Here's how the part is built. I have some questions about the finished solid (model axes, mm). A direction names the side the tool comes from. Give positions to 0.01 mm unless a question says otherwise; leave off trailing zeros. Loops run counter-clockwise (first coordinate to the right, second up) from the corner with the lowest first, then second, coordinate; pieces in that order, holes last. Notation, with made-up numbers: (-7, 42) - (46, 42) arc R18 cw to (46, 55) - close; hole circle Ø6 at (35, 70.5). An arc over 180 degrees is marked (long way). Use one line per item in the form item = value.
from build123d import *

# Parameters (mm, degrees)
F0_R     = 2.2923424458
F1_DEPTH = 3


with BuildPart() as f1:
    # F0 (on Top) → F1 (new body)
    with BuildSketch(Plane.XY):
        with BuildLine():
            ThreePointArc((-10.2711248099, 20.5369088401), (-7.4915699128, 20.9637629982), (-4.6818986464, 21.0815648356))
            ThreePointArc((-4.6818986464, 21.0815648356), (-3.8272791749, 22.4288026174), (-3.528424334, 23.9960007114))
            ThreePointArc((-3.528424334, 23.9960007114), (-9.7309143278, 27.7851076735), (-10.2711248099, 20.5369088401))
        make_face()
        with Locations((-7.7870538317, 23.9960007114)):
            Circle(F0_R, mode=Mode.SUBTRACT)
        with BuildLine():
            ThreePointArc((-10.2711248099, 20.5369088401), (-7.3740175906, 19.7574483332), (-4.6818986464, 21.0815648356))
            ThreePointArc((-4.6818986464, 21.0815648356), (-7.4915699128, 20.9637629982), (-10.2711248099, 20.5369088401))
        make_face()
        with BuildLine():
            ThreePointArc((17.6210584616, 7.2744961396), (-14.3609161452, -12.5373076401), (9.5862937371, 16.4779539925))
            ThreePointArc((9.5862937371, 16.4779539925), (2.7986315485, 19.8534789731), (-4.6818986464, 21.0815648356))
            ThreePointArc((-4.6818986464, 21.0815648356), (-7.3740175906, 19.7574483332), (-10.2711248099, 20.5369088401))
            ThreePointArc((-10.2711248099, 20.5369088401), (-15.9577589353, -27.3838876789), (17.6210584616, 7.2744961396))
        make_face()
        with BuildLine():
            ThreePointArc((19.3017870188, -6.0611376539), (-21.9723847969, -20.9981833276), (-5.4997475818, 19.687499851))
            ThreePointArc((-5.4997475818, 19.687499851), (-10.7496275746, 17.4612976364), (-15.179797656, 13.870920318))
            Line((-15.179797656, 13.870920318), (-15.6238832555, 13.3781558918))
            ThreePointArc((-15.6238832555, 13.3781558918), (-16.1982928509, 12.6896602283), (-16.7419419606, 11.9766256516))
            Line((-16.7419419606, 11.9766256516), (-17.2084446119, 11.3084951626))
            ThreePointArc((-17.2084446119, 11.3084951626), (-18.814029944, 8.43031492), (-19.9359758104, 5.3314339541))
            Line((-19.9359758104, 5.3314339541), (-20.2770843766, 3.8746306645))
            ThreePointArc((-20.2770843766, 3.8746306645), (-5.2009908425, -19.8687278573), (19.3017870188, -6.0611376539))
        make_face(mode=Mode.SUBTRACT)
    extrude(amount=F1_DEPTH)


solid = f1.part
(1) If we section it at D-D (x = -13.5): List the corners of the cut face in (y, z) for me.
Geometry says:
outline = (-28.4, 0) - (-26.67, 0) - (-26.67, 3) - (-28.4, 3) - close; (-15.58, 0) - (-13.46, 0) - (-13.46, 3) - (-15.58, 3) - close; (13.46, 0) - (15.48, 0) - (15.48, 3) - (13.46, 3) - close; (18.02, 0) - (19.63, 0) - (19.63, 3) - (18.02, 3) - close
(2) If I drill on probe 1 along X at (y, z) = (-4.5, 0.3); probe 2 along Y at (x, z) = (0, 1.05); probe 3 along Y at (x, z) = (2, 0.2), over which ranges is the centre line in solid material (lowest first)?
Geometry says:
probe_1 = -30.49 to -28.69, -20.17 to -18.52, 18.52 to 20.45
probe_2 = -29.35 to -27.9, -20.48 to -19.06, 19.06 to 20.58
probe_3 = -28.86 to -27.41, -20.36 to -18.96, 18.96 to 20.1
(3) Thinking about a two-plate mould opening in Y: for faces 1 (the cylindrical face through (-13.86, -13.09, 1.48)), 2 (the flat face through (-18, -7, 0)), 3 (the cylindrical face through (-5.62, -19.76, 1.48)), which applies, pulls with the +Y half, pulls with the -Y half, needs draft (parallel to the pull), parting line crosses it, or undercut?
Geometry says:
face_1 = undercut
face_2 = needs draft
face_3 = undercut
(4) If we section it at B-B (x = 5.5): List the corners of the cut face in (y, z) for me, plus the area to 3 significant figures.
Geometry says:
outline = (-27.58, 0) - (-26.1, 0) - (-26.1, 3) - (-27.58, 3) - close; (-19.66, 0) - (-18.25, 0) - (-18.25, 3) - (-19.66, 3) - close; (18.25, 0) - (18.81, 0) - (18.81, 3) - (18.25, 3) - close
area = 10.3 mm²
(5) If we section it at C-C (z = 1.75): List the corners of the cut face in (x, y) for me.
Geometry says:
outline = (-10.27, 20.54) arc R25.47 ccw (long way) to (17.62, 7.27) arc R19.06 cw (long way) to (9.59, 16.48) arc R25.47 ccw to (-4.68, 21.08) arc R4.26 ccw (long way) to start; hole (-20.28, 3.87) - (-19.94, 5.33) arc R20.43 cw to (-17.21, 11.31) - (-16.74, 11.98) arc R20.43 cw to (-15.62, 13.38) - (-15.18, 13.87) arc R20.43 cw to (-5.5, 19.69) arc R24.03 ccw (long way) to (19.3, -6.06) arc R20.43 cw to start; hole circle Ø4.58 at (-7.79, 24)
(6) If we section it at A-A (y = 0): List the corners of the cut face in (x, z) for me.
Geometry says:
outline = (-30.11, 0) - (-28.3, 0) - (-28.3, 3) - (-30.11, 3) - close; (-20.66, 0) - (-19.06, 0) - (-19.06, 3) - (-20.66, 3) - close; (19.06, 0) - (20.07, 0) - (20.07, 3) - (19.06, 3) - close
(7) For faces 4 (the flat face through (-18, -7, 3)), 5 (the flat face through (-20.104, 4.613, 1.479)), which set-ups out of +Z, -Z, +X, -X, +Y, -Y let a thin tool reach every point of the face, with its end or its side?
Geometry says:
face_4 = +Z, +X, -X, +Y, -Y
face_5 = +Z, -Z
(8) For P1, Ø1, axis at x = 7, z = 1, coming from the +Y side, with a flat end and sliding along its axis, tell me the tip position at first contact or that it passes through.
Geometry says:
P1 = 18.33
